from build123d import *

# Parameters (mm, degrees)
SKETCH1_R           = 40.9
SKETCH1_R_2         = 39.5
BOSS_EXTRUDE1_DEPTH = 145
SKETCH1_3_R         = 42.5
SKETCH1_3_R_2       = 40.9
BOSS_EXTRUDE2_DEPTH = 55


with BuildPart() as part:
    # Sketch1 → Boss-Extrude1 (new, symmetric)
    with BuildSketch(Plane(origin=(0, 0, 0), x_dir=(1, 0, 0), z_dir=(0, 1, 0))):
        Circle(SKETCH1_R)
        Circle(SKETCH1_R_2, mode=Mode.SUBTRACT)
    extrude(amount=BOSS_EXTRUDE1_DEPTH, both=True)

    # Sketch1<3> → Boss-Extrude2 (add, symmetric)
    with BuildSketch(Plane(origin=(0, 0, 0), x_dir=(1, 0, 0), z_dir=(0, 1, 0))):
        Circle(SKETCH1_3_R)
        Circle(SKETCH1_3_R_2, mode=Mode.SUBTRACT)
    extrude(amount=BOSS_EXTRUDE2_DEPTH, both=True)


solid = part.part
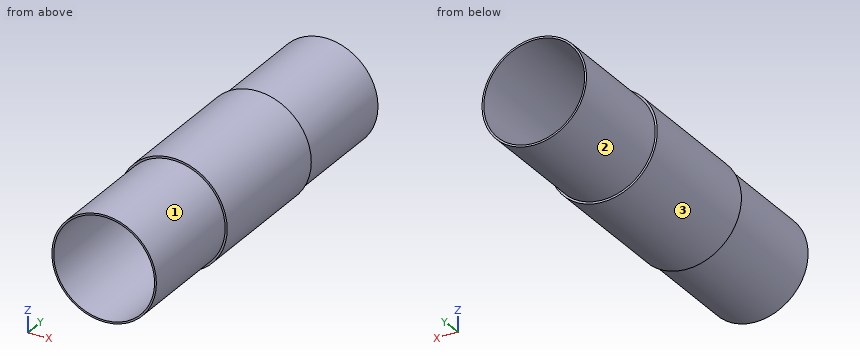
For this review, take the finished solid that the model builds, in its own axes (mm). Face numbers are marked on the shaded views. A direction names the side the tool comes from. Round coordinates to 2 decimals unless told otherwise and drop trailing zeros. Write each loop counter-clockwise with the first axis right and the second up, starting at its lowest first coordinate (ties: lowest second). Pieces come first, ordered by that corner, then holes. Notation, with made-up numbers: (69, 83) - (85, 83) arc R11 cw to (85, 103) - close; hole circle Ø10 at (-27.75, 31). An arc over 180 degrees is marked (long way). Use a Markdown table: item, result.
Q1. We need section D-D (y = 82). Give the boundary of the cut face in (x, z), plus the area to 3 significant figures.
Derived:
| item | result |
|---|---|
| outline | circle Ø81.8 at (0, 0); hole circle Ø79 at (0, 0) |
| area | 354 mm2 |
Q2. Clearance check with flat-ended pins moving along their axes: pin 1 (5 mm diameter, centred on x = -22.5, y = 110, fed in from -Z); pin 2 (1.5 mm diameter, centred on x = -28, y = -107, fed in from -Z); pin 3 (1 mm diameter, centred on x = -17, y = 47.5, fed in from -Z). State where each tip first meets the part, or that it passes through.
Derived:
| item | result |
|---|---|
| pin 1 | stops at z = -35.68 |
| pin 2 | stops at z = -30.5 |
| pin 3 | stops at z = -39.17 |
Q3. Wall thickness on line 1 along Z through (x, y) = (0, 0.5); line 2 along X through (y, z) = (-62, 0): over which ranges is each line inside the solid? List them lowest first.
Derived:
| item | result |
|---|---|
| line 1 | z = -42.5 to -39.5, 39.5 to 42.5 |
| line 2 | x = -40.9 to -39.5, 39.5 to 40.9 |
Q4. We need section A-A (x = 0). Give the boundary of the cut face in (y, z).
Derived:
| item | result |
|---|---|
| outline | (-145, -40.9) - (-55, -40.9) - (-55, -42.5) - (55, -42.5) - (55, -40.9) - (145, -40.9) - (145, -39.5) - (-145, -39.5) - close; (-145, 39.5) - (145, 39.5) - (145, 40.9) - (55, 40.9) - (55, 42.5) - (-55, 42.5) - (-55, 40.9) - (-145, 40.9) - close |
Q5. Machinability: for the marked faces 1, 2 and 3, which of the approach directions +Z, -Z, +X, -X, +Y, -Y give a long, thin tool a straight path to every point of the face, cutting with its end or side? Answer none if there is none.
Derived:
| item | result |
|---|---|
| face 1 | -Y |
| face 2 | +Y |
| face 3 | +Y, -Y |
Q6. We need section B-B (z = 0). Give the boundary of the cut face in (x, y), plus the area to 3 significant figures.
Derived:
| item | result |
|---|---|
| outline | (-42.5, -55) - (-40.9, -55) - (-40.9, -145) - (-39.5, -145) - (-39.5, 145) - (-40.9, 145) - (-40.9, 55) - (-42.5, 55) - close; (39.5, -145) - (40.9, -145) - (40.9, -55) - (42.5, -55) - (42.5, 55) - (40.9, 55) - (40.9, 145) - (39.5, 145) - close |
| area | 1,160 mm2 |
Q7. We need section C-C (y = -13.5). Give the boundary of the cut face in (x, z), plus the area to 3 significant figures.
Derived:
| item | result |
|---|---|
| outline | circle Ø85 at (0, 0); hole circle Ø79 at (0, 0) |
| area | 773 mm2 |
